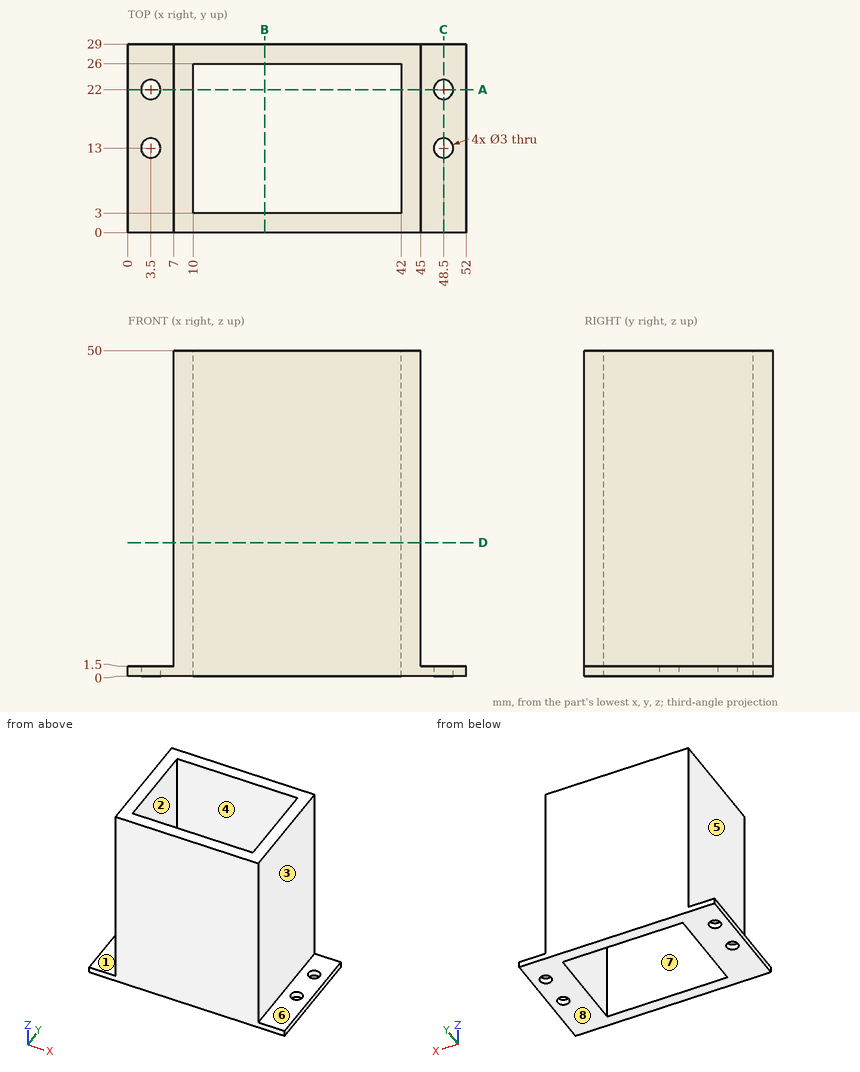
Part print with two shaded views. Sizes in mm from the minimum x, y, z corner. A direction names the side the tool comes from. Coordinates: 2 decimals unless noted, no trailing zeros. Write each loop counter-clockwise with the first axis right and the second up, starting at its lowest first coordinate (ties: lowest second). Pieces come first, ordered by that corner, then holes. Notation, with made-up numbers: (-33.75, -8.5) - (-6.75, -8.5) arc R5 cw to (-6.75, -3.5) - close; hole circle Ø7 at (37.5, 18). An arc over 180 degrees is marked (long way). Use a Markdown table: item, result. Add a question column.
Item 1: Band-saw the part on A-A, the plane y = 22. Write the cut outline in (x, z), and give its area (3 significant figures).
Item 2: Drop flat-ended pins along their axis: pin 1 (3.5 mm diameter, centred on x = 48.5, y = 22, fed in from +Z); pin 2 (1.8 mm diameter, centred on x = 3.5, y = 22, fed in from +Z); pin 3 (12 mm diameter, centred on y = 19.5, z = 9.5, fed in from +X); pin 4 (10 mm diameter, centred on y = 15.5, z = 11.5, fed in from -X). Give the stop position or say it passes through.
Item 3: Drill centre lines: line 1 along Y through (x, z) = (48.5, 0.9); line 2 along X through (y, z) = (12.25, 25); line 3 along Y through (x, z) = (11, 30). Where is each one in solid material? Low to high.
Item 4: Two-plate mould, pull along X, no slides. Class the marked faces 1, 2, 3 and 4: pulls with the +X half, pulls with the -X half, needs draft (parallel to the pull), parting line crosses it, or undercut.
Item 5: Band-saw the part on D-D, the plane z = 20.5. Write the cut outline in (x, y).
Item 6: 3-axis set-ups, long thin cutter, end or side, ignore diameter. For the marked faces 5, 6, 7 and 8: which of +Z, -Z, +X, -X, +Y, -Y reach the whole face in a straight line?
Item 7: Band-saw the part on B-B, the plane x = 21. Write the cut outline in (y, z), and give its area (3 significant figures).
Item 8: Band-saw the part on C-C, the plane x = 48.5. Write the cut outline in (y, z), and give its area (3 significant figures).
A:
| question | item | result |
|---|---|---|
| 1 | outline | (0, 0) - (2, 0) - (2, 1.5) - (0, 1.5) - close; (5, 0) - (10, 0) - (10, 50) - (7, 50) - (7, 1.5) - (5, 1.5) - close; (42, 0) - (47, 0) - (47, 1.5) - (45, 1.5) - (45, 50) - (42, 50) - close; (50, 0) - (52, 0) - (52, 1.5) - (50, 1.5) - close |
| 1 | area | 312 mm² |
| 2 | pin 1 | stops at z = 1.5 |
| 2 | pin 2 | passes through |
| 2 | pin 3 | stops at x = 45 |
| 2 | pin 4 | stops at x = 7 |
| 3 | line 1 | y = 0 to 11.5, 14.5 to 20.5, 23.5 to 29 |
| 3 | line 2 | x = 7 to 10, 42 to 45 |
| 3 | line 3 | y = 0 to 3, 26 to 29 |
| 4 | face 1 | needs draft |
| 4 | face 2 | undercut |
| 4 | face 3 | pulls with the +X half |
| 4 | face 4 | undercut |
| 5 | outline | (7, 0) - (45, 0) - (45, 29) - (7, 29) - close; hole (10, 3) - (42, 3) - (42, 26) - (10, 26) - close |
| 6 | face 5 | +Z, -X, +Y, -Y |
| 6 | face 6 | +Z, +X, +Y, -Y |
| 6 | face 7 | +Z, -Z |
| 6 | face 8 | -Z, +X, -X, +Y, -Y |
| 7 | outline | (0, 0) - (3, 0) - (3, 50) - (0, 50) - close; (26, 0) - (29, 0) - (29, 50) - (26, 50) - close |
| 7 | area | 300 mm² |
| 8 | outline | (0, 0) - (11.5, 0) - (11.5, 1.5) - (0, 1.5) - close; (14.5, 0) - (20.5, 0) - (20.5, 1.5) - (14.5, 1.5) - close; (23.5, 0) - (29, 0) - (29, 1.5) - (23.5, 1.5) - close |
| 8 | area | 34.5 mm² |
